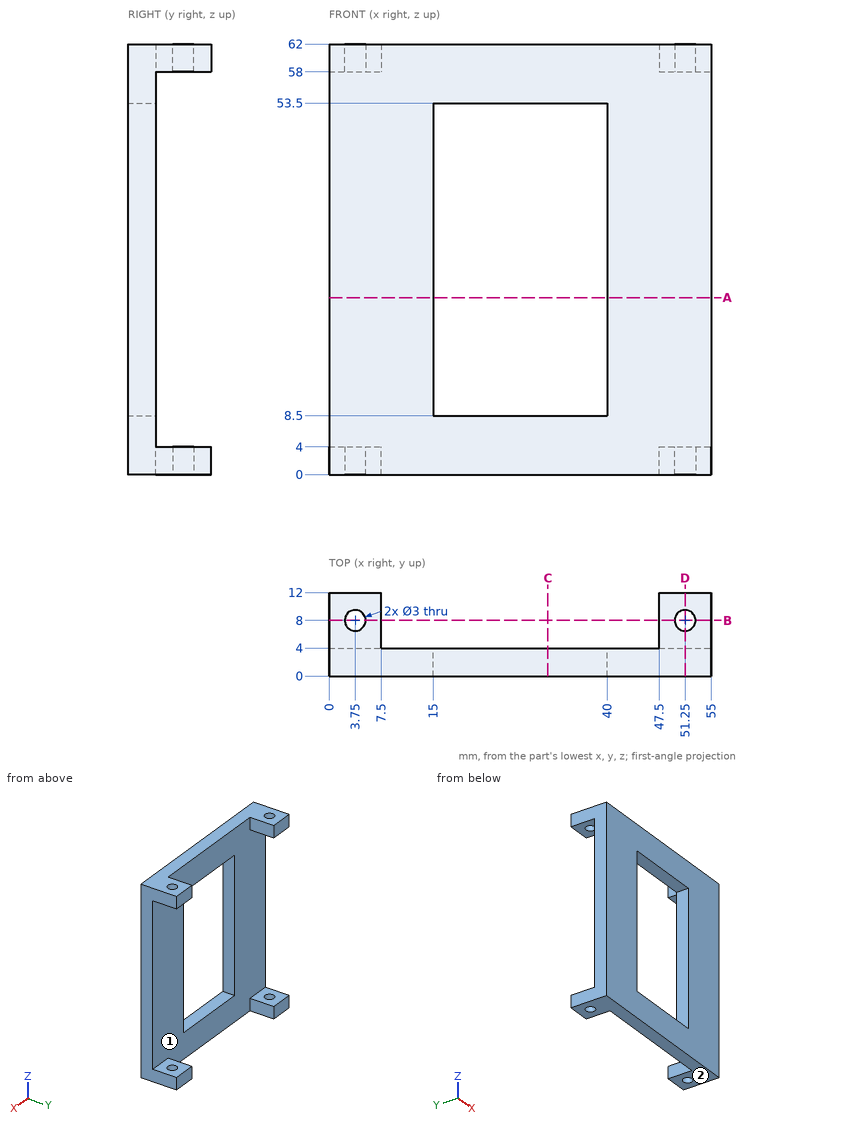
For this review, use the dimensioned drawing (mm, ordinates from the lowest corner) and the shaded views. Give positions to 0.01 mm unless a question says otherwise; leave off trailing zeros. Write each loop counter-clockwise with the first axis right and the second up, starting at its lowest first coordinate (ties: lowest second). Pieces come first, ordered by that corner, then holes. Notation, with made-up numbers: M 86,49 L 111,49 A28 ccw 111,73 Z; hole C -14,8.25 d4. An arc over 180 degrees is marked long. Answer as a JSON object with one key per item and string values. Group by question number.
Item 1: Consider section D-D on x = 51.25. Write out the cut boundary in (y, z).
Item 2: For probe 1 along X at (y, z) = (2, 47.5); probe 2 along Z at (x, y) = (23.5, 0.5); probe 3 along Y at (x, z) = (3.75, 61.1), list the stretches that pass through material, from the lowest coordinate up. Write a range as [from, to].
Item 3: Draft analysis for pull direction X (two halves, no side actions). For the marked faces 1 and 2, state which applies: +X half, -X half, draft (parallel to the pull), parting line (faces both ways), or undercut.
Item 4: Consider section B-B on y = 8. Count the separate pieces of the cut face and the enclosed holes in it, plus the area to 3 significant figures.
Item 5: Consider section A-A on z = 25.5. Write out the cut boundary in (x, y).
Item 6: For pin 1 Ø12 at (x, z) = (18.5, 37) entering from +Y; pin 2 Ø2.5 at (x, y) = (51.25, 8) entering from -Z, all flat-tipped, find the tip position at first contact; note any pin that passes through.
Item 7: Consider section C-C on x = 31.5. Write out the cut boundary in (y, z).
Check result:
{
 "1": {"outline": "M 0,0 L 6.5,0 L 6.5,4 L 4,4 L 4,58 L 6.5,58 L 6.5,62 L 0,62 Z; M 9.5,0 L 12,0 L 12,4 L 9.5,4 Z; M 9.5,58 L 12,58 L 12,62 L 9.5,62 Z"},
 "2": {"probe 1": "x = [0, 15], [40, 55]", "probe 2": "z = [0, 8.5], [53.5, 62]", "probe 3": "y = [0, 6.5], [9.5, 12]"},
 "3": {"face 1": "undercut", "face 2": "draft"},
 "4": {"separate pieces": "8", "enclosed holes": "0", "area": "72.0 mm^2"},
 "5": {"outline": "M 0,0 L 15,0 L 15,4 L 0,4 Z; M 40,0 L 55,0 L 55,4 L 40,4 Z"},
 "6": {"pin 1": "stops at y = 4", "pin 2": "passes through"},
 "7": {"outline": "M 0,0 L 4,0 L 4,8.5 L 0,8.5 Z; M 0,53.5 L 4,53.5 L 4,62 L 0,62 Z"}
}
